from build123d import *

# Parameters (mm, degrees)
SKETCH_1_R      = 1.875
EXTRUDE_1_DEPTH = 1.6
SKETCH_1_3_W    = 19.6
SKETCH_1_3_H    = 10.5
EXTRUDE_2_DEPTH = 5


with BuildPart() as part:
    # Sketch 1 → Extrude 1 (new body)
    with BuildSketch(Plane(origin=(0, 0, 0), x_dir=(1, 0, 0), z_dir=(0, 1, 0))):
        Polygon((-7.103957265, -14.564899143), (-9.405761269, -12.314899143), (-9.405761269, -5.514899143), (10.194238731, -5.514899143), (10.194238731, -12.314899143), (7.996042735, -14.564899143), align=None)
        with Locations(Location((0.446042735, -11.789899143, 0), (0, 0, 270))):
            Circle(SKETCH_1_R, mode=Mode.SUBTRACT)
    extrude(amount=EXTRUDE_1_DEPTH)

    # Sketch 1_3 → Extrude 2 (add)
    with BuildSketch(Plane(origin=(0, 0, 0), x_dir=(1, 0, 0), z_dir=(0, 1, 0))):
        with Locations((0.394238731, -0.264899143)):
            Rectangle(SKETCH_1_3_W, SKETCH_1_3_H)
    extrude(amount=EXTRUDE_2_DEPTH)


solid = part.part
The listing builds one solid part. Answer for the finished solid, in the listing's coordinates (mm). A direction names the side the tool comes from. Give positions to 0.01 mm unless a question says otherwise; leave off trailing zeros. Write each loop counter-clockwise with the first axis right and the second up, starting at its lowest first coordinate (ties: lowest second). Pieces come first, ordered by that corner, then holes. Notation, with made-up numbers: (-34, 17.25) - (-20, 17.25) arc R30 cw to (-20, 56.25) - close; hole circle Ø2 at (79.25, 60.5). An arc over 180 degrees is marked (long way). Use a Markdown table: item, result.
1. Each of these flat-tipped pins is pushed along its axis until it touches: P1, Ø4.5, axis at x = 0.5, z = 9, coming from the +Y side; P2, Ø3.5, axis at x = 0.45, z = 11.79, coming from the -Y side. Where does it stop, or does it pass through?
Values follow:
| item | result |
|---|---|
| P1 | stops at y = 1.6 |
| P2 | passes through |
2. A tool of negligible diameter and unlimited length cuts with its end or side. For faces 5 (the flat face through (0, 3, 5.515)), 6 (the flat face through (0, 0, 5)), from which of +Z, -Z, +X, -X, +Y, -Y can it reach the whole face along a straight path? Write none if from no direction.
Values follow:
| item | result |
|---|---|
| face 5 | +Z, +X, -X, +Y |
| face 6 | +Z, -Z, +X, -X, -Y |
3. Section C-C on x = -4.5 is taken. Write down the section's boundary in (y, z).
Values follow:
| item | result |
|---|---|
| outline | (0, -4.99) - (5, -4.99) - (5, 5.51) - (1.6, 5.51) - (1.6, 14.56) - (0, 14.56) - close |
4. Section D-D on y = 0.75 is taken. Write down the section's boundary in (x, z) (3 decimals), plus the area to 3 significant figures.
Values follow:
| item | result |
|---|---|
| outline | (-9.406, -4.985) - (10.194, -4.985) - (10.194, 12.315) - (7.996, 14.565) - (-7.104, 14.565) - (-9.406, 12.315) - close; hole circle Ø3.75 at (0.446, 11.79) |
| area | 367 mm² |
5. For a pull along Z with two mould halves and no side action, classify faces 1 (the flat face through (0, 2, -4.985)), 2 (the cylindrical face through (-0.272, 0.789, 13.522)), 3 (the flat face through (9.111, 0.789, 13.424)), 4 (the flat face through (0, 5, 0)) as released by +Z, released by -Z, zero draft, split by the parting line, or undercut.
Values follow:
| item | result |
|---|---|
| face 1 | released by -Z |
| face 2 | undercut |
| face 3 | released by +Z |
| face 4 | zero draft |
6. Section B-B on z = 13.25 is taken. Write down the section's boundary in (x, y).
Values follow:
| item | result |
|---|---|
| outline | (-8.45, 0) - (-0.73, 0) - (-0.73, 1.6) - (-8.45, 1.6) - close; (1.62, 0) - (9.28, 0) - (9.28, 1.6) - (1.62, 1.6) - close |
7. Find the intervals of material crossed by probe 1 along Z at (x, y) = (5, 2.25); probe 2 along X at (y, z) = (1.35, 12.25); probe 3 along Y at (x, z) = (-8, 10), in increasing order. Write a range as from..to.
Values follow:
| item | result |
|---|---|
| probe 1 | z = -4.99..5.51 |
| probe 2 | x = -9.41..-1.37, 2.26..10.19 |
| probe 3 | y = 0..1.6 |
8. Section A-A on x = -0.25 is taken. Write down the section's boundary in (y, z).
Values follow:
| item | result |
|---|---|
| outline | (0, -4.99) - (5, -4.99) - (5, 5.51) - (1.6, 5.51) - (1.6, 10.05) - (0, 10.05) - close; (0, 13.53) - (1.6, 13.53) - (1.6, 14.56) - (0, 14.56) - close |
